from build123d import *

# Parameters (mm, degrees)
CORTAR_EXTRUIR1_DEPTH = 3.5
REDONDEO1_R           = 0.8


with BuildPart() as part:
    # Croquis1 → Revolución1 (revolve)
    with BuildSketch(Plane(origin=(0, 0, 0), x_dir=(0, 0, -1), z_dir=(1, 0, 0))):
        Polygon((0, 2.5), (-55, 2.5), (-55, 5.5), (-51.5, 5.5), (-51.5, 6), (-55, 6), (-55, 9.5), (-51.5, 9.5), (-51.5, 11), (-47.5, 11), (-47.5, 8.5), (0, 8.5), align=None)
    revolve(axis=Axis((0, 0, 58.146951639), (0, 0, -1)))

    # Croquis2 → Cortar-Extruir1 (cut)
    with BuildSketch(Plane.XY.offset(55)):
        with BuildLine():
            Line((-5, 0), (-5, 8.077747211))
            ThreePointArc((-5, 8.077747211), (0, -9.5), (5, 8.077747211))
            Line((5, 8.077747211), (5, 0))
            Line((5, 0), (5, -2.291287847))
            ThreePointArc((5, -2.291287847), (0, -5.5), (-5, -2.291287847))
            Line((-5, -2.291287847), (-5, 0))
        make_face()
    extrude(amount=-CORTAR_EXTRUIR1_DEPTH, mode=Mode.SUBTRACT)

    # Redondeo1
    redondeo1_edges = [part.edges().sort_by_distance(p)[0] for p in [
        (0, 9.5, 55),
        (0, 6, 55),
        (5, 5.697186001, 55),
        (-5, 5.697186001, 55),
    ]]
    fillet(redondeo1_edges, radius=REDONDEO1_R)

    # Simetría1: part across plane


with BuildPart() as part_1:
    add(part.part)
    add(part.part.mirror(Plane.XY))


solid = part_1.part
Model file for the job. Use its own axes, mm. A direction names the side the tool comes from. Round coordinates to 2 decimals unless told otherwise and drop trailing zeros. Order: outer loops, then holes, each group sorted by start corner. A loop starts at its lowest first (then second) coordinate and runs counter-clockwise, first axis right, second up. Notation, with made-up numbers: M 61.5,14 L 115.5,14 A27 cw 115.5,47 Z; hole C -22,20.5 d9. An arc over 180 degrees is marked long. Write each question's results on one line, items separated by ' | '. Start each with the question number.
(1) Which spindle directions (+Z, -Z, +X, -X, +Y, -Y) get a long thin tool onto all of the face, cutting with end or side? Do faces 1 (the face through (-8.1, 3.2, 47.5)), 2 (the face through (-0.1, 9.5, 52.8)), 3 (the face through (5, 0, 53)), 4 (the face through (-5, 0, 53)). Say none if no direction does.
(2) Saw through at C-C, the plane x = 6.5. Give the cut face in (y, z).
(3) Probe probe 1 along Z at (x, y) = (6, -8.75); probe 2 along X at (y, z) = (0, 6.5); probe 3 along Y at (x, z) = (-1.25, 8.5). List the from-to ranges inside material, lowest first. Write a range as from..to.
(4) Saw through at B-B, the plane z = -3.5. Give the cut face in (x, y), then the cut area to 3 significant figures.
(5) Drop flat-ended pins along their axis: pin 1 (1.8 mm diameter, centred on y = 0.5, z = 53, fed in from +X); pin 2 (12 mm diameter, centred on x = -7, z = -2.5, fed in from +Y); pin 3 (2 mm diameter, centred on y = -7, z = -37, fed in from -X). Give the stop position or say it passes through.
(6) Two-plate mould, pull along Y, no slides. Class faces 5 (the face through (5, 0, -53)), 6 (the face through (0, 6, -53)), 7 (the face through (-0.1, 9.5, -52.8)), 8 (the face through (0, 6, 53)): pulls with the +Y half, pulls with the -Y half, needs draft (parallel to the pull), parting line crosses it, or undercut.
(7) Saw through at D-D, the plane y = -7. Give the cut face in (x, z), then the cut area to 3 significant figures.
(8) Saw through at A-A, the plane y = 0. Give the cut face in (x, z).
Established:
1) face 1: none | face 2: +Z, +Y | face 3: +Z, +X, +Y, -Y | face 4: +Z, -X, +Y, -Y
2) outline: M -8.87,-51.5 L 8.87,-51.5 L 8.87,-47.5 L 5.48,-47.5 L 5.48,47.5 L 8.87,47.5 L 8.87,51.5 L -8.87,51.5 L -8.87,47.5 L -5.48,47.5 L -5.48,-47.5 L -8.87,-47.5 Z
3) probe 1: z = -51.5..-47.5, 47.5..51.5 | probe 2: x = -8.5..-2.5, 2.5..8.5 | probe 3: y = -8.41..-2.17, 2.17..8.41
4) outline: C 0,0 d17; hole C 0,0 d5 | area: 207 mm^2
5) pin 1: stops at x = 5 | pin 2: stops at y = 8.44 | pin 3: stops at x = -6.02
6) face 5: needs draft | face 6: undercut | face 7: pulls with the +Y half | face 8: undercut
7) outline: M -8.49,-51.5 L 8.49,-51.5 L 8.49,-47.5 L 4.82,-47.5 L 4.82,47.5 L 8.49,47.5 L 8.49,51.5 L -8.49,51.5 L -8.49,47.5 L -4.82,47.5 L -4.82,-47.5 L -8.49,-47.5 Z | area: 1,050 mm^2
8) outline: M -11,-51.5 L -5,-51.5 L -5,-55 L -2.5,-55 L -2.5,55 L -5,55 L -5,51.5 L -11,51.5 L -11,47.5 L -8.5,47.5 L -8.5,-47.5 L -11,-47.5 Z; M 2.5,-55 L 5,-55 L 5,-51.5 L 11,-51.5 L 11,-47.5 L 8.5,-47.5 L 8.5,47.5 L 11,47.5 L 11,51.5 L 5,51.5 L 5,55 L 2.5,55 Z
